The listing builds one solid part. Answer for the finished solid, in the listing's coordinates (mm). A direction names the side the tool comes from. Round coordinates to 2 decimals unless told otherwise and drop trailing zeros. Write each loop counter-clockwise with the first axis right and the second up, starting at its lowest first coordinate (ties: lowest second). Pieces come first, ordered by that corner, then holes. Notation, with made-up numbers: M 16,-32.5 L 68,-32.5 A15 cw 68,-15.5 Z; hole C 58.5,-27 d5. An arc over 180 degrees is marked long. Answer as CSV lines item,"result". Start each with the question number.
Autodesk Inventor part; units mm, degrees
ref_plane "YZ Plane" through (0, 0, 0) normal (1, 0, 0) x (0, 1, 0)
ref_plane "XZ Plane" through (0, 0, 0) normal (0, 1, 0) x (-1, 0, 0)
ref_plane "XY Plane" through (0, 0, 0) normal (0, 0, 1) x (1, 0, 0)
sketch "Sketch1" plane through (0, 0, 0) normal (0, 0, 1) x (1, 0, 0)
  arc A0 (-1.5, -1.3229) -> (-1.5, 1.3229) centre (0, 0) ccw
  line L0 (-1.5, 1.3229) -> (-1.5, -1.3229)
  circle A1 centre (0, 0) radius 70
  dimension "d0" = 4
  dimension "d1" = 1.5
  dimension "d2" = 140
extrude "Extrusion1" add sketch "Sketch1" along normal blind 6
sketch "Sketch2" plane through (0, 0, 0) normal (0, 0, -1) x (-1, 0, 0)
  circle A0 centre (0, 0) radius 70 construction
  arc A1 (1.5, 1.3229) -> (1.5, -1.3229) centre (0, 0) ccw construction
  circle A2 centre (0, 0) radius 70
  line L0 (1.5, -1.3229) -> (1.5, 1.3229) construction
  arc A3 (1.5, 1.3229) -> (1.5, -1.3229) centre (0, 0) ccw construction
  line L1 (0, 0) -> (-1.5321, 1.2856)
  arc A4 (55, 0) -> (42.1324, 35.3533) centre (0, 0) ccw
  line L2 (0, 0) -> (1.5, 0) construction
  line L3 (25, 0) -> (55, 0) construction
  line L4 (0, 0) -> (1.5, 1.2586)
  line L5 (19.1511, 16.0697) -> (42.1324, 35.3533)
  line L6 (0, 0) -> (1.5, 0) construction
  line L7 (25, 0) -> (55, 0) construction
  line L8 (0, 0) -> (1.5, 0)
  line L9 (25, 0) -> (70, 0)
  line L10 (55, 0) -> (25, 0)
  line L11 (-9.902, 22.9554) -> (-21.7844, 50.5019)
  line L12 (15.7742, 52.6894) -> (7.1701, 23.9497)
  arc A5 (15.7742, 52.6894) -> (-21.7844, 50.5019) centre (0, 0) ccw
  line L13 (-24.831, -2.9023) -> (-54.6281, -6.3851)
  line L14 (-45.9518, 30.223) -> (-20.8872, 13.7377)
  arc A6 (-45.9518, 30.223) -> (-54.6281, -6.3851) centre (0, 0) ccw
  line L15 (-4.3412, -24.6202) -> (-9.5506, -54.1644)
  line L16 (-42.1324, -35.3533) -> (-19.1511, -16.0697)
  arc A7 (-42.1324, -35.3533) -> (-9.5506, -54.1644) centre (0, 0) ccw
  arc A8 (-19.1511, -16.0697) -> (-4.3412, -24.6202) centre (0, 0) ccw
  arc A9 (-20.8872, 13.7377) -> (-24.831, -2.9023) centre (0, 0) ccw
  arc A10 (25, 0) -> (19.1511, 16.0697) centre (0, 0) ccw
  arc A11 (7.1701, 23.9497) -> (-9.902, 22.9554) centre (0, 0) ccw
  dimension "d10" = 110
  dimension "d13" = 220
extrude "Extrusion4" cut sketch "Sketch2" against normal through all contours L9 A10 L5 A4 | L11 A5 L12 A11 | L13 A6 L14 A9 | L15 A7 L16 A8
properties part number "back_cir_hold2"
Q1. Find section C-C (x = 15.5). Determine the outline of the cut face in (y, z).
Q2. Find section B-B (y = -31). Determine the outline of the cut face in (x, z).
Q3. Find section A-A (z = 1.7). Determine the outline of the cut face in (x, y).
Q4. Find section D-D (y = 10). Determine the outline of the cut face in (x, z), plus the area to 3 significant figures.
Q5. For faces 1 (the face through (-1, -15, 0)), 2 (the face through (39.52, -4.62, 2.96)), determine the directions among +Z, -Z, +X, -X, +Y, -Y from which every point of the face is accessible in a straight line to the end or side of a thin tool.
Q6. Straight lines are drawn through the part: L1, parallel to Y at x = 0, z = 1.55; L2, parallel to Y at x = 30, z = 2.05; L3, parallel to X at y = -1.5, z = 5.15. For each, find the intervals that lie inside material, in ascending order.
Q7. The mould has two halves that part along X. Classify faces 3 (the face through (-23.534, 8.436, 2.958)), 4 (the face through (-1, -15, 6)), 5 (the face through (-55.55, 42.594, 2.958)): +X half, -X half, draft (parallel to the pull), parting line (faces both ways), or undercut.
Q8. This flat-tipped pin is pushed along its axis until it touches: P1, Ø1.5, axis at x = -1.5, z = 5, coming from the -Y side. Where does it stop, or does it pass through?
Reported:
1,outline,"M -68.26,0 L -52.77,0 L -52.77,6 L -68.26,6 Z; M -19.62,0 L 35.93,0 L 35.93,6 L -19.62,6 Z; M 52.77,0 L 68.26,0 L 68.26,6 L 52.77,6 Z"
2,outline,"M -62.76,0 L 5.47,0 L 5.47,6 L -62.76,6 Z; M 36.94,0 L 62.76,0 L 62.76,6 L 36.94,6 Z"
3,outline,"C 0,0 d140; hole M -55,0 L -25,0 A25 cw -19.15,16.07 L -42.13,35.35 A55 ccw Z; hole M -15.77,52.69 L -7.17,23.95 A25 cw 9.9,22.96 L 21.78,50.5 A55 ccw Z; hole M -1.5,-1.32 A2 ccw long -1.5,1.32 Z; hole M 4.34,-24.62 L 9.55,-54.16 A55 ccw 42.13,-35.35 L 19.15,-16.07 A25 cw Z; hole M 20.89,13.74 A25 cw 24.83,-2.9 L 54.63,-6.39 A55 ccw 45.95,30.22 Z"
4,outline,"M -69.28,0 L -54.08,0 L -54.08,6 L -69.28,6 Z; M -22.91,0 L 22.91,0 L 22.91,6 L -22.91,6 Z; M 54.08,0 L 69.28,0 L 69.28,6 L 54.08,6 Z"
4,area,"457 mm2"
5,face 1,"-Z, +X, -X, +Y, -Y"
5,face 2,"+Z, -Z"
6,L1,"y = -70 to -2, 2 to 25, 55 to 70"
6,L2,"y = -63.25 to -46.1, -25.17 to -3.51, 19.73 to 63.25"
6,L3,"x = -69.98 to -1.32, 1.32 to 24.95, 54.98 to 69.98"
7,face 3,"undercut"
7,face 4,"draft"
7,face 5,"parting line"
8,P1,"stops at y = -70"
